Verification items for the finished model (mm, model axes). A direction names the side the tool comes from. Give positions to 0.01 mm unless a question says otherwise; leave off trailing zeros. Write each loop counter-clockwise with the first axis right and the second up, starting at its lowest first coordinate (ties: lowest second). Pieces come first, ordered by that corner, then holes. Notation, with made-up numbers: (44, 87) - (49, 87) arc R22 ccw to (49, 96) - close; hole circle Ø4 at (-31, -35.5). An arc over 180 degrees is marked (long way). Put each result on its own line as item: value.
from build123d import *

# Parameters (mm, degrees)
SKETCH1_W           = 16.2205508
SKETCH1_H           = 16.7068193
BOSS_EXTRUDE1_DEPTH = 5.25
SKETCH2_W           = 16.2205508
SKETCH2_H           = 16.7068193
SKETCH2_R           = 3.25
BOSS_EXTRUDE2_DEPTH = 3
BOSS_EXTRUDE3_START = -3
SKETCH1_3_W         = 16.2205508
SKETCH1_3_H         = 16.7068193
SKETCH1_3_R         = 3.25
BOSS_EXTRUDE3_DEPTH = 3


with BuildPart() as part:
    # Sketch1 → Boss-Extrude1 (new body)
    with BuildSketch(Plane.XY):
        Rectangle(SKETCH1_W, SKETCH1_H)
        Polygon((3.127313958, -5.416666667), (6.254627916, 0), (3.127313958, 5.416666667), (-3.127313958, 5.416666667), (-6.254627916, 0), (-3.127313958, -5.416666667), align=None, mode=Mode.SUBTRACT)
    extrude(amount=BOSS_EXTRUDE1_DEPTH)

    # Sketch2 → Boss-Extrude2 (add)
    with BuildSketch(Plane.XY.offset(5.25)):
        Rectangle(SKETCH2_W, SKETCH2_H)
        Circle(SKETCH2_R, mode=Mode.SUBTRACT)
    extrude(amount=BOSS_EXTRUDE2_DEPTH)

    # Sketch1_3 → Boss-Extrude3 (add)
    # profile 1 of 2: a face of its own
    with BuildSketch(Plane.XY.offset(BOSS_EXTRUDE3_START)):
        Rectangle(SKETCH1_3_W, SKETCH1_3_H)
        Polygon((3.127313958, -5.416666667), (6.254627916, 0), (3.127313958, 5.416666667), (-3.127313958, 5.416666667), (-6.254627916, 0), (-3.127313958, -5.416666667), align=None, mode=Mode.SUBTRACT)
    # profile 2 of 2: a face of its own
    with BuildSketch(Plane.XY.offset(BOSS_EXTRUDE3_START)):
        Polygon((-3.127313958, -5.416666667), (3.127313958, -5.416666667), (6.254627916, 0), (3.127313958, 5.416666667), (-3.127313958, 5.416666667), (-6.254627916, 0), align=None)
        Circle(SKETCH1_3_R, mode=Mode.SUBTRACT)
    extrude(amount=BOSS_EXTRUDE3_DEPTH)


solid = part.part
Q1. Section check C-C, the plane z = 4.25. Record the cut outline in (x, y), plus the area to 3 significant figures.
Answers follow:
outline: (-8.11, -8.35) - (8.11, -8.35) - (8.11, 8.35) - (-8.11, 8.35) - close; hole (-6.25, 0) - (-3.13, -5.42) - (3.13, -5.42) - (6.25, 0) - (3.13, 5.42) - (-3.13, 5.42) - close
area: 169 mm2
Q2. Set-up check for faces 1 (the face through (0, 8.353, 3)), 2 (the face through (3, -2, 0)): record each of +Z, -Z, +X, -X, +Y, -Y from which the full face is reachable in a straight line by a thin tool's end or side.
Answers follow:
face 1: +Z, -Z, +X, -X, +Y
face 2: none
Q3. Section check A-A, the plane x = 0. Record the cut outline in (y, z).
Answers follow:
outline: (-8.35, -3) - (-3.25, -3) - (-3.25, 0) - (-5.42, 0) - (-5.42, 5.25) - (-3.25, 5.25) - (-3.25, 8.25) - (-8.35, 8.25) - close; (3.25, -3) - (8.35, -3) - (8.35, 8.25) - (3.25, 8.25) - (3.25, 5.25) - (5.42, 5.25) - (5.42, 0) - (3.25, 0) - close
Q4. Release check for a two-part mould opening along Z. For faces 3 (the face through (-8.11, 0, 3)), 4 (the face through (3.5, 0.1, -3)), 5 (the face through (-4.713, -2.67, 2.588)), 6 (the face through (-4.669, 2.746, 2.588)) record: released by +Z, released by -Z, zero draft, split by the parting line, or undercut.
Answers follow:
face 3: zero draft
face 4: released by -Z
face 5: undercut
face 6: undercut
Q5. Section check B-B, the plane y = 1.75. Record the cut outline in (x, z).
Answers follow:
outline: (-8.11, -3) - (-2.74, -3) - (-2.74, 0) - (-5.24, 0) - (-5.24, 5.25) - (-2.74, 5.25) - (-2.74, 8.25) - (-8.11, 8.25) - close; (2.74, -3) - (8.11, -3) - (8.11, 8.25) - (2.74, 8.25) - (2.74, 5.25) - (5.24, 5.25) - (5.24, 0) - (2.74, 0) - close
Q6. Scan lines: line 1 along Z through (x, y) = (-2, 4.5); line 2 along Y through (x, z) = (0, 6.4); line 3 along X through (y, z) = (1, 3.25). Record each from-to range of solid material in increasing order.
Answers follow:
line 1: z = -3 to 0, 5.25 to 8.25
line 2: y = -8.35 to -3.25, 3.25 to 8.35
line 3: x = -8.11 to -5.68, 5.68 to 8.11
Q7. Section check D-D, the plane y = -3.5. Record the cut outline in (x, z).
Answers follow:
outline: (-8.11, -3) - (8.11, -3) - (8.11, 8.25) - (-8.11, 8.25) - close; hole (-4.23, 0) - (4.23, 0) - (4.23, 5.25) - (-4.23, 5.25) - close
